from build123d import *

# Parameters (mm, degrees)
EXTRUDE_1_DEPTH = 1100
OTHER_1_DEPTH   = 58


# Read off the part's stored shape, not the designer's step: Полость1
with BuildPart() as part:
    # Эскиз1 → Бобышка-Вытянуть1 (new body)
    with BuildSketch(Plane.XY):
        with BuildLine():
            Line((0, -140), (0, 0))
            Line((0, 0), (58, 0))
            Line((58, 0), (58, -1.9))
            ThreePointArc((58, -1.9), (57.121320344, -4.021320344), (55, -4.9))
            Line((55, -4.9), (12.9, -4.9))
            ThreePointArc((12.9, -4.9), (7.243145751, -7.243145751), (4.9, -12.9))
            Line((4.9, -12.9), (4.9, -127.1))
            ThreePointArc((4.9, -127.1), (7.243145751, -132.756854249), (12.9, -135.1))
            Line((12.9, -135.1), (55, -135.1))
            ThreePointArc((55, -135.1), (57.121320344, -135.978679656), (58, -138.1))
            Line((58, -138.1), (58, -140))
            Line((58, -140), (0, -140))
        make_face()
    extrude(amount=-EXTRUDE_1_DEPTH)

    # Полость1 outline → Полость1 (cut)
    with BuildSketch(Plane.YZ):
        with BuildLine():
            Line((-140, 0), (-140, -58))
            Line((-140, -58), (-138.1, -58))
            ThreePointArc((-138.1, -58), (-135.978679656, -57.121320344), (-135.1, -55))
            Line((-135.1, -55), (-135.1, -12.9))
            ThreePointArc((-135.1, -12.9), (-132.756854249, -7.243145751), (-127.1, -4.9))
            Line((-127.1, -4.9), (-12.9, -4.9))
            ThreePointArc((-12.9, -4.9), (-7.243145751, -7.243145751), (-4.9, -12.9))
            Line((-4.9, -12.9), (-4.9, -55))
            ThreePointArc((-4.9, -55), (-4.021320344, -57.121320344), (-1.9, -58))
            Line((-1.9, -58), (0, -58))
            Line((0, -58), (0, 0))
            Line((0, 0), (-140, 0))
        make_face()
    extrude(amount=OTHER_1_DEPTH, mode=Mode.SUBTRACT)


solid = part.part
Can you work these out from the model? Positions are in its coordinate system, mm. A direction names the side the tool comes from. Give positions to 0.01 mm unless a question says otherwise; leave off trailing zeros. Loops run counter-clockwise (first coordinate to the right, second up) from the corner with the lowest first, then second, coordinate; pieces in that order, holes last. Notation, with made-up numbers: M 85.5,-13.5 L 128.5,-13.5 A20 ccw 128.5,24.5 Z; hole C 38.5,-29 d4. An arc over 180 degrees is marked long. One line per item, written item: value. Start each with the question number.
1) I'm going to push flat-ended pins straight in: pin 1 (3 mm diameter, centred on y = -104.5, z = -438.5, fed in from +X); pin 2 (5 mm diameter, centred on x = 16, z = -826, fed in from +Y); pin 3 (2 mm diameter, centred on x = 15, y = -1.5, fed in from +Z); pin 4 (14 mm diameter, centred on x = 4.5, z = -34.5, fed in from +Y). Where does each tip first touch, or does it pass through?
2) On a 3-axis mill with a long thin cutter (end or side, diameter ignored), from which of +Z, -Z, +X, -X, +Y, -Y can I reach the whole of each face in a straight line? I mean faces 1 (the face through (3, -75, -1100)), 2 (the face through (4.9, -69, -545)). Say none if no direction works.
3) If we section it at B-B, the plane z = -528: Write out the boundary of the cut face in (x, y), and give its area (3 significant figures).
4) If we section it at C-C, the plane y = -64.5: Write out the boundary of the cut face in (x, z).
5) If I drill on line 1 (Y direction, x = 39, z = -208.5); line 2 (X direction, y = -108, z = -277.5); line 3 (Y direction, x = 6, z = -477), over which ranges is the centre line in solid material (lowest first)? Write a range as [from, to].
6) Thinking about a two-plate mould opening in Y: for faces 3 (the face through (29, -140, -572)), 4 (the face through (34, -135.1, -570)), 5 (the face through (29, 0, -572)), which applies, +Y half, -Y half, draft (parallel to the pull), parting line (faces both ways), or undercut?
7) If we section it at A-A, the plane x = 32: Write out the boundary of the cut face in (y, z).
Completed:
1. pin 1: stops at x = 4.9
1. pin 2: stops at y = 0
1. pin 3: stops at z = -57.94
1. pin 4: stops at y = -4.9
2. face 1: -Z, +X, -X, +Y, -Y
2. face 2: +Z, -Z, +X
3. outline: M 0,-140 L 58,-140 L 58,-138.1 A3 ccw 55,-135.1 L 12.9,-135.1 A8 cw 4.9,-127.1 L 4.9,-12.9 A8 cw 12.9,-4.9 L 55,-4.9 A3 ccw 58,-1.9 L 58,0 L 0,0 Z
3. area: 1,230 mm^2
4. outline: M 0,-1100 L 4.9,-1100 L 4.9,-4.9 L 0,-4.9 Z
5. line 1: y = [-140, -135.1], [-4.9, 0]
5. line 2: x = [0, 4.9]
5. line 3: y = [-140, -131.15], [-8.85, 0]
6. face 3: -Y half
6. face 4: undercut
6. face 5: +Y half
7. outline: M -140,-1100 L -135.1,-1100 L -135.1,-55 A3 cw -138.1,-58 L -140,-58 Z; M -4.9,-1100 L 0,-1100 L 0,-58 L -1.9,-58 A3 cw -4.9,-55 Z
